Can you work these out from the model? Positions are in its coordinate system, mm. Round coordinates to 2 decimals unless told otherwise and drop trailing zeros. Loops run counter-clockwise (first coordinate to the right, second up) from the corner with the lowest first, then second, coordinate; pieces in that order, holes last.
(1) If I drill on line 1 along Z through (x, y) = (7.5, 5); line 2 along X through (y, z) = (7.25, 85); line 3 along X through (y, z) = (1.5, 165.5), over which ranges is the centre line in solid material (lowest first)?
(2) I want a section at A-A on z = 139. Write out the boundary of the cut face in (x, y), plus the area to 3 significant figures.
(3) I want a section at B-B on y = 5. Give the number of separate pieces and of enclosed holes in the cut face, plus the area to 3 significant figures.
(4) Will these pins go through, and if not, where does the flat tip stop? pin 1 Ø2 at (y, z) = (4, 61) entering from -X; pin 2 Ø2 at (y, z) = (5.5, 101) entering from -X; pin 3 Ø1.2 at (y, z) = (5.5, 131) entering from +X.
Solid Edge part; units mm, degrees
sketch "Sketch1" plane through (0, 0, 0) normal (0, -1, 0) x (1, 0, 0)
  line L0 (-98.417, 1.7127) -> (11.583, 1.7127)
  line L1 (11.583, 1.7127) -> (11.583, 181.7127)
  line L2 (11.583, 181.7127) -> (-98.417, 181.7127)
  line L3 (-98.417, 181.7127) -> (-98.417, 1.7127)
  dimension "D1" = 98.417
  dimension "D2" = 98.417
extrude "Protrusion1" add sketch "Sketch1" against normal blind 10
sketch "Sketch2" plane through (-48.417, 0, 81.7127) normal (0, -1, 0) x (1, 0, 0)
  circle A0 centre (-36.5, 86.5) radius 5
  circle A1 centre (46.5, 86.5) radius 5
  circle A2 centre (-36.5, 3.5) radius 5
  circle A3 centre (46.5, 3.5) radius 5
  circle A4 centre (5, 45) radius 15
extrude "Cutout1" cut sketch "Sketch2" against normal through all
extrude "Cutout2" [suppressed]
extrude "Protrusion2" [suppressed]
extrude "Cutout3" [suppressed]
hole "Hole_1" at (11.583, 5, 61.7127) direction (-1, 0, 0) diameter 4.134 depth 20 thread major 5 thread length 2
hole "Hole1" at (11.583, 5, 101.7127) direction (-1, 0, 0) diameter 4.134 depth 20 thread major 5 thread length 2
hole "Hole2" at (11.583, 5, 21.7127) direction (-1, 0, 0) diameter 4.134 depth 20 thread major 5 thread length 2
hole "Hole3" at (11.583, 5, 131.7127) direction (-1, 0, 0) diameter 4.134 depth 20 thread major 5 thread length 2
mirror "Mirror1" about plane through (-43.417, 5, 91.7127) normal (1, 0, 0) of "Hole_1", "Hole1", "Hole2", "Hole3"
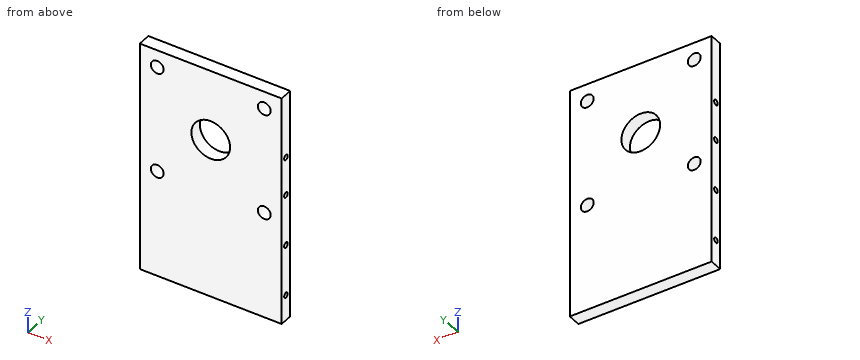
Filled sheet:
1. line 1: z = 1.71 to 19.65, 23.78 to 59.65, 63.78 to 99.65, 103.78 to 129.65, 133.78 to 181.71
1. line 2: x = -98.42 to -89.91, -79.92 to -6.91, 3.08 to 11.58
1. line 3: x = -98.42 to -89.12, -80.72 to -6.12, 2.28 to 11.58
2. outline: (-98.42, 0) - (-52.02, 0) - (-52.02, 10) - (-98.42, 10) - close; (-34.81, 0) - (11.58, 0) - (11.58, 10) - (-34.81, 10) - close
2. area: 928 mm2
3. separate pieces: 1
3. enclosed holes: 5
3. area: 18,100 mm2
4. pin 1: stops at x = -98.42
4. pin 2: stops at x = -78.42
4. pin 3: stops at x = -8.42
